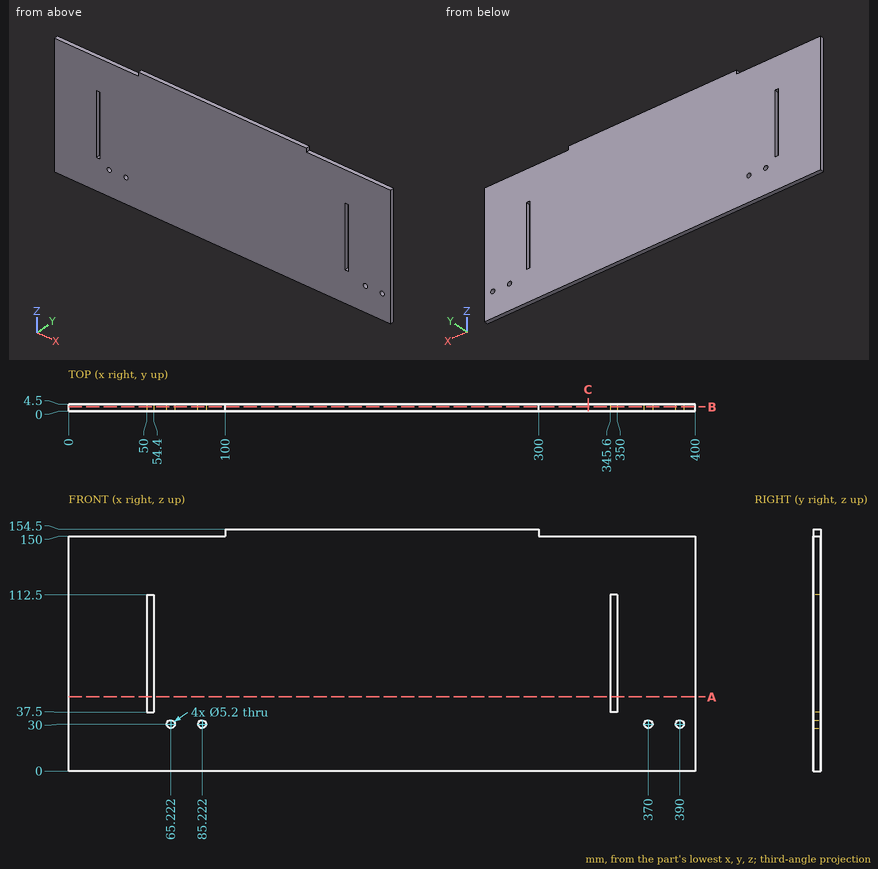
Answer from the drawing. Dimensions are ordinates in mm from the lowest x, y and z of the part. Give positions to 0.01 mm unless a question says otherwise; leave off trailing zeros. Write each loop counter-clockwise with the first axis right and the second up, starting at its lowest first coordinate (ties: lowest second). Pieces come first, ordered by that corner, then holes. Notation, with made-up numbers: (-33.75, -10.75) - (-12.75, -10.75) arc R21 cw to (-12.75, 21.25) - close; hole circle Ø10 at (13.5, 15). An arc over 180 degrees is marked (long way). One line per item, written item: value. Start each with the question number.
1. Find section C-C (x = 331.5). Write down the section's boundary in (y, z).
2. Find section A-A (z = 47.5). Write down the section's boundary in (x, y).
3. Given pin 1 (2 mm diameter, centred on x = 347, y = 1.5, fed in from +Z), flat-ended and moving along its own axis, determine where the tip first touches the part or whether it passes through.
4. Find section B-B (y = 2.7). Write down the section's boundary in (x, z).
5. Consider probe 1 along X at (y, z) = (4.15, 88); probe 2 along X at (y, z) = (1.8, 30); probe 3 along Z at (x, y) = (370, 0.9). Determine where each line is inside the solid, lowest interval first.
Geometry results:
1. outline: (0, 0) - (4.5, 0) - (4.5, 150) - (0, 150) - close
2. outline: (0, 0) - (50, 0) - (50, 4.5) - (0, 4.5) - close; (54.4, 0) - (345.6, 0) - (345.6, 4.5) - (54.4, 4.5) - close; (350, 0) - (400, 0) - (400, 4.5) - (350, 4.5) - close
3. pin 1: z = 150
4. outline: (0, 0) - (400, 0) - (400, 150) - (300, 150) - (300, 154.5) - (100, 154.5) - (100, 150) - (0, 150) - close; hole (50, 37.5) - (54.4, 37.5) - (54.4, 112.5) - (50, 112.5) - close; hole circle Ø5.2 at (65.22, 30); hole circle Ø5.2 at (85.22, 30); hole (345.6, 37.5) - (350, 37.5) - (350, 112.5) - (345.6, 112.5) - close; hole circle Ø5.2 at (370, 30); hole circle Ø5.2 at (390, 30)
5. probe 1: 0 to 50, 54.4 to 345.6, 350 to 400
5. probe 2: 0 to 62.62, 67.82 to 82.62, 87.82 to 367.4, 372.6 to 387.4, 392.6 to 400
5. probe 3: 0 to 27.4, 32.6 to 150
